from build123d import *

# Parameters (mm, degrees)
BOSS_EXTRUDE1_DEPTH     = 12.7
M5_SHAFT_REACH          = 14.7
SKETCH2_W               = 12.7
SKETCH2_H               = 5.400000122
M5_START                = -12.7
SKETCH3_W               = 4.1
SKETCH3_H               = 8.15
M5_NUT_DEPTH            = 12.7
RASBERRY_PI_HOLES_REACH = 14.7
SKETCH5_R               = 1.625


with BuildPart() as part:
    # Sketch1 → Boss-Extrude1 (new body)
    with BuildSketch(Plane.XY):
        Polygon((194.31, -63.5), (-194.31, -63.5), (-194.31, -38.1), (-207.01, -38.1), (-207.01, 38.1), (-194.31, 38.1), (-194.31, 63.5), (194.31, 63.5), (194.31, 38.1), (207.01, 38.1), (207.01, -38.1), (194.31, -38.1), align=None)
    extrude(amount=BOSS_EXTRUDE1_DEPTH)

    # Sketch2 → m5 shaft (cut, up to next)
    with BuildSketch(Plane.XY.offset(12.7), mode=Mode.PRIVATE) as m5_shaft_sk1:
        with Locations((-187.96, 50.8)):
            Rectangle(SKETCH2_W, SKETCH2_H)
    m5_shaft_tool1 = extrude(m5_shaft_sk1.sketch, amount=-M5_SHAFT_REACH, mode=Mode.PRIVATE) & part.part
    add(m5_shaft_tool1.solids().sort_by_distance((-187.96, 50.8, 12.7))[0], mode=Mode.SUBTRACT)
    # Sketch2 → m5 shaft (cut, up to next)
    with BuildSketch(Plane.XY.offset(12.7), mode=Mode.PRIVATE) as m5_shaft_sk2:
        with Locations((-187.96, -50.8)):
            Rectangle(SKETCH2_W, SKETCH2_H)
    m5_shaft_tool2 = extrude(m5_shaft_sk2.sketch, amount=-M5_SHAFT_REACH, mode=Mode.PRIVATE) & part.part
    add(m5_shaft_tool2.solids().sort_by_distance((-187.96, -50.8, 12.7))[0], mode=Mode.SUBTRACT)
    # Sketch2 → m5 shaft (cut, up to next)
    with BuildSketch(Plane.XY.offset(12.7), mode=Mode.PRIVATE) as m5_shaft_sk3:
        with Locations((187.96, -50.8)):
            Rectangle(SKETCH2_W, SKETCH2_H)
    m5_shaft_tool3 = extrude(m5_shaft_sk3.sketch, amount=-M5_SHAFT_REACH, mode=Mode.PRIVATE) & part.part
    add(m5_shaft_tool3.solids().sort_by_distance((187.96, -50.8, 12.7))[0], mode=Mode.SUBTRACT)
    # Sketch2 → m5 shaft (cut, up to next)
    with BuildSketch(Plane.XY.offset(12.7), mode=Mode.PRIVATE) as m5_shaft_sk4:
        with Locations((187.96, 50.8)):
            Rectangle(SKETCH2_W, SKETCH2_H)
    m5_shaft_tool4 = extrude(m5_shaft_sk4.sketch, amount=-M5_SHAFT_REACH, mode=Mode.PRIVATE) & part.part
    add(m5_shaft_tool4.solids().sort_by_distance((187.96, 50.8, 12.7))[0], mode=Mode.SUBTRACT)

    # Sketch3 → m5 nut (cut)
    with BuildSketch(Plane.XY.offset(12.7).offset(M5_START)):
        with Locations((-186.31, 50.8)):
            Rectangle(SKETCH3_W, SKETCH3_H)
        with Locations((-186.31, -50.8)):
            Rectangle(SKETCH3_W, SKETCH3_H)
        with Locations((186.31, -50.8)):
            Rectangle(SKETCH3_W, SKETCH3_H)
        with Locations((186.31, 50.8)):
            Rectangle(SKETCH3_W, SKETCH3_H)
    extrude(amount=M5_NUT_DEPTH, mode=Mode.SUBTRACT)

    # Sketch5 → rasberry pi holes (cut, up to next)
    with BuildSketch(Plane.XY.offset(12.7), mode=Mode.PRIVATE) as rasberry_pi_holes_sk1:
        with Locations((-142.61, 19)):
            Circle(SKETCH5_R)
    rasberry_pi_holes_tool1 = extrude(rasberry_pi_holes_sk1.sketch, amount=-RASBERRY_PI_HOLES_REACH, mode=Mode.PRIVATE) & part.part
    add(rasberry_pi_holes_tool1.solids().sort_by_distance((-142.61, 19, 12.7))[0], mode=Mode.SUBTRACT)
    # Sketch5 → rasberry pi holes (cut, up to next)
    with BuildSketch(Plane.XY.offset(12.7), mode=Mode.PRIVATE) as rasberry_pi_holes_sk2:
        with Locations((-93.61, 19)):
            Circle(SKETCH5_R)
    rasberry_pi_holes_tool2 = extrude(rasberry_pi_holes_sk2.sketch, amount=-RASBERRY_PI_HOLES_REACH, mode=Mode.PRIVATE) & part.part
    add(rasberry_pi_holes_tool2.solids().sort_by_distance((-93.61, 19, 12.7))[0], mode=Mode.SUBTRACT)
    # Sketch5 → rasberry pi holes (cut, up to next)
    with BuildSketch(Plane.XY.offset(12.7), mode=Mode.PRIVATE) as rasberry_pi_holes_sk3:
        with Locations((-93.61, -39)):
            Circle(SKETCH5_R)
    rasberry_pi_holes_tool3 = extrude(rasberry_pi_holes_sk3.sketch, amount=-RASBERRY_PI_HOLES_REACH, mode=Mode.PRIVATE) & part.part
    add(rasberry_pi_holes_tool3.solids().sort_by_distance((-93.61, -39, 12.7))[0], mode=Mode.SUBTRACT)
    # Sketch5 → rasberry pi holes (cut, up to next)
    with BuildSketch(Plane.XY.offset(12.7), mode=Mode.PRIVATE) as rasberry_pi_holes_sk4:
        with Locations((-142.61, -39)):
            Circle(SKETCH5_R)
    rasberry_pi_holes_tool4 = extrude(rasberry_pi_holes_sk4.sketch, amount=-RASBERRY_PI_HOLES_REACH, mode=Mode.PRIVATE) & part.part
    add(rasberry_pi_holes_tool4.solids().sort_by_distance((-142.61, -39, 12.7))[0], mode=Mode.SUBTRACT)
    # Sketch5 → rasberry pi holes (cut, up to next)
    with BuildSketch(Plane.XY.offset(12.7), mode=Mode.PRIVATE) as rasberry_pi_holes_sk5:
        with Locations((142.61, -39)):
            Circle(SKETCH5_R)
    rasberry_pi_holes_tool5 = extrude(rasberry_pi_holes_sk5.sketch, amount=-RASBERRY_PI_HOLES_REACH, mode=Mode.PRIVATE) & part.part
    add(rasberry_pi_holes_tool5.solids().sort_by_distance((142.61, -39, 12.7))[0], mode=Mode.SUBTRACT)
    # Sketch5 → rasberry pi holes (cut, up to next)
    with BuildSketch(Plane.XY.offset(12.7), mode=Mode.PRIVATE) as rasberry_pi_holes_sk6:
        with Locations((93.61, -39)):
            Circle(SKETCH5_R)
    rasberry_pi_holes_tool6 = extrude(rasberry_pi_holes_sk6.sketch, amount=-RASBERRY_PI_HOLES_REACH, mode=Mode.PRIVATE) & part.part
    add(rasberry_pi_holes_tool6.solids().sort_by_distance((93.61, -39, 12.7))[0], mode=Mode.SUBTRACT)
    # Sketch5 → rasberry pi holes (cut, up to next)
    with BuildSketch(Plane.XY.offset(12.7), mode=Mode.PRIVATE) as rasberry_pi_holes_sk7:
        with Locations((93.61, 19)):
            Circle(SKETCH5_R)
    rasberry_pi_holes_tool7 = extrude(rasberry_pi_holes_sk7.sketch, amount=-RASBERRY_PI_HOLES_REACH, mode=Mode.PRIVATE) & part.part
    add(rasberry_pi_holes_tool7.solids().sort_by_distance((93.61, 19, 12.7))[0], mode=Mode.SUBTRACT)
    # Sketch5 → rasberry pi holes (cut, up to next)
    with BuildSketch(Plane.XY.offset(12.7), mode=Mode.PRIVATE) as rasberry_pi_holes_sk8:
        with Locations((142.61, 19)):
            Circle(SKETCH5_R)
    rasberry_pi_holes_tool8 = extrude(rasberry_pi_holes_sk8.sketch, amount=-RASBERRY_PI_HOLES_REACH, mode=Mode.PRIVATE) & part.part
    add(rasberry_pi_holes_tool8.solids().sort_by_distance((142.61, 19, 12.7))[0], mode=Mode.SUBTRACT)


solid = part.part
For this review, take the finished solid that the model builds, in its own axes (mm). A direction names the side the tool comes from. Give positions to 0.01 mm unless a question says otherwise; leave off trailing zeros. One line per question, with ' | ' between items.
1) Insertion check: pin 1 Ø4 at (x, z) = (198, 5.5) entering from -Y; pin 2 Ø4 at (y, z) = (-49, 2) entering from +X; pin 3 Ø2.5 at (y, z) = (-51.5, 7.5) entering from +X. Each pin has a flat end and moves straight along its axis. Give the tip position at first contact, or say it passes through.
Resolved:
pin 1: stops at y = -38.1 | pin 2: stops at x = 194.31 | pin 3: stops at x = 181.61
2) To check wall thickness, follow probe 1 along Y at (x, z) = (-142.61, 7.5) (3 decimals); probe 2 along X at (y, z) = (47, 8); probe 3 along X at (y, z) = (51, 3.75). State the ranges of each line that lie inside material, in increasing order.
Resolved:
probe 1: y = -63.5 to -40.625, -37.375 to 17.375, 20.625 to 63.5 | probe 2: x = -194.31 to -188.36, -184.26 to 184.26, 188.36 to 194.31 | probe 3: x = -181.61 to 181.61
3) We need section A-A (z = 6). Give the number of separate pieces and of enclosed holes in the cut face, plus the area to 3 significant figures.
Resolved:
separate pieces: 1 | enclosed holes: 8 | area: 50,900 mm2
4) For faces 1 (the flat face through (-207.01, -1, 6)), 2 (the flat face through (-194.31, -59, 6)), 3 (the flat face through (194.31, 59, 6)), 4 (the flat face through (201, -38.1, 6)), 5 (the flat face through (-201, 38.1, 6)), list the 3-axis set-ups (+Z, -Z, +X, -X, +Y, -Y) from which the entire face can be reached by the end or side of a thin tool; tool diameter is ignored.
Resolved:
face 1: +Z, -Z, -X, +Y, -Y | face 2: +Z, -Z, -X, -Y | face 3: +Z, -Z, +X, +Y | face 4: +Z, -Z, +X, -Y | face 5: +Z, -Z, -X, +Y
